Work out the finished part from the listing and answer in its coordinate system (mm). Face numbers are marked on the shaded views. A direction names the side the tool comes from. Give positions to 0.01 mm unless a question says otherwise; leave off trailing zeros. Loops run counter-clockwise (first coordinate to the right, second up) from the corner with the lowest first, then second, coordinate; pieces in that order, holes last. Notation, with made-up numbers: (0, 31) - (24, 31) arc R9 cw to (24, 46) - close; hole circle Ø5 at (74.25, -17). An arc over 180 degrees is marked (long way). Use CSV: the item, a comma, the result in double quotes.
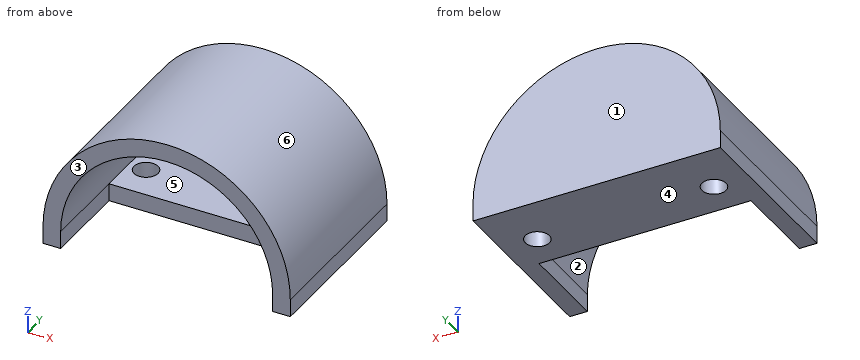
from build123d import *

# Parameters (mm, degrees)
SKETCH1_W           = 88.9
SKETCH1_H           = 25.4
SKETCH1_R           = 4.3561
BOSS_EXTRUDE1_DEPTH = 6.35
SKETCH2_W           = 88.9
SKETCH2_H           = 6.35
BOSS_EXTRUDE2_DEPTH = 6.35
BOSS_EXTRUDE3_START = -63.5
BOSS_EXTRUDE3_DEPTH = 63.5


with BuildPart() as part:
    # Sketch1 → Boss-Extrude1 (new body)
    with BuildSketch(Plane.XY):
        Rectangle(SKETCH1_W, SKETCH1_H)
        with Locations((-31.75, 0)):
            Circle(SKETCH1_R, mode=Mode.SUBTRACT)
        with Locations((31.75, 0)):
            Circle(SKETCH1_R, mode=Mode.SUBTRACT)
    extrude(amount=BOSS_EXTRUDE1_DEPTH)

    # Sketch2 → Boss-Extrude2 (add)
    with BuildSketch(Plane(origin=(0, 12.7, 0), x_dir=(1, 0, 0), z_dir=(0, 1, 0))):
        with Locations((0, -3.175)):
            Rectangle(SKETCH2_W, SKETCH2_H)
        with BuildLine():
            ThreePointArc((-44.45, -6.35), (0, -50.8), (44.45, -6.35))
            Line((44.45, -6.35), (-44.45, -6.35))
        make_face()
    extrude(amount=BOSS_EXTRUDE2_DEPTH)

    # Sketch3 → Boss-Extrude3 (add)
    with BuildSketch(Plane(origin=(0, 19.05, 0), x_dir=(1, 0, 0), z_dir=(0, 1, 0)).offset(BOSS_EXTRUDE3_START)):
        with BuildLine():
            ThreePointArc((-44.45, -6.35), (0, -50.8), (44.45, -6.35))
            Line((44.45, -6.35), (44.45, 0))
            Line((44.45, 0), (38.1, 0))
            Line((38.1, 0), (38.1, -6.35))
            ThreePointArc((38.1, -6.35), (0, -44.45), (-38.1, -6.35))
            Line((-38.1, -6.35), (-38.1, 0))
            Line((-38.1, 0), (-44.45, 0))
            Line((-44.45, 0), (-44.45, -6.35))
        make_face()
    extrude(amount=BOSS_EXTRUDE3_DEPTH)


solid = part.part
Item 1: For the marked faces 1 and 2, determine the directions among +Z, -Z, +X, -X, +Y, -Y from which every point of the face is accessible in a straight line to the end or side of a thin tool.
Determined:
face 1,"+Z, -Z, +X, -X, +Y"
face 2,"-Y"
Item 2: A cutting plane is placed at C-C on z = 12.5. Determine the outline of the cut face in (x, y), and give its area (3 significant figures).
Determined:
outline,"(-44.02, -44.45) - (-37.6, -44.45) - (-37.6, 12.7) - (37.6, 12.7) - (37.6, -44.45) - (44.02, -44.45) - (44.02, 19.05) - (-44.02, 19.05) - close"
area,"1,290 mm²"
Item 3: Given P1, Ø2, axis at y = -38, z = 16, coming from the +X side; P2, Ø7.5, axis at x = 0.5, y = -1, coming from the +Z side; P3, Ø11.5, axis at x = -16, z = 33, coming from the -Y side, each flat-ended and moving along its own axis, determine where each tip first touches the part or whether it passes through.
Determined:
P1,"stops at x = 43.6"
P2,"stops at z = 50.8"
P3,"stops at y = 12.7"
Item 4: Find the intervals of material crossed by line 1 (X direction, y = -23.5, z = 41.5); line 2 (X direction, y = -40, z = 10); line 3 (Y direction, x = -29, z = 31), in increasing order.
Determined:
line 1,"x = -27.21 to -14.7, 14.7 to 27.21"
line 2,"x = -44.3 to -37.92, 37.92 to 44.3"
line 3,"y = 12.7 to 19.05"
Item 5: The mould has two halves that part along Z. Classify the marked faces 3, 4, 5 and 6: pulls with the +Z half, pulls with the -Z half, needs draft (parallel to the pull), parting line crosses it, or undercut.
Determined:
face 3,"needs draft"
face 4,"pulls with the -Z half"
face 5,"undercut"
face 6,"pulls with the +Z half"
Item 6: A cutting plane is placed at A-A on y = 0. Determine the outline of the cut face in (x, z), and give its area (3 significant figures).
Determined:
outline,"(-44.45, 0) - (-36.11, 0) - (-36.11, 6.35) - (-38.1, 6.35) arc R38.1 cw to (38.1, 6.35) - (36.11, 6.35) - (36.11, 0) - (44.45, 0) - (44.45, 6.35) arc R44.45 ccw to (-44.45, 6.35) - close; (-27.39, 0) - (27.39, 0) - (27.39, 6.35) - (-27.39, 6.35) - close"
area,"1,280 mm²"
Item 7: A cutting plane is placed at B-B on y = 9. Determine the outline of the cut face in (x, z), and give its area (3 significant figures).
Determined:
outline,"(-44.45, 0) - (44.45, 0) - (44.45, 6.35) arc R44.45 ccw to (-44.45, 6.35) - close; hole (-38.1, 6.35) - (38.1, 6.35) arc R38.1 ccw to start"
area,"1,390 mm²"
Item 8: A cutting plane is placed at D-D on x = 0. Determine the outline of the cut face in (y, z), and give its area (3 significant figures).
Determined:
outline,"(-44.45, 44.45) - (12.7, 44.45) - (12.7, 6.35) - (-12.7, 6.35) - (-12.7, 0) - (19.05, 0) - (19.05, 50.8) - (-44.45, 50.8) - close"
area,"847 mm²"
